Design review of the part built by this model. Coordinates are the model's own, in mm. Face numbers are marked on the shaded views. A direction names the side the tool comes from. Give positions to 0.01 mm unless a question says otherwise; leave off trailing zeros. Write each loop counter-clockwise with the first axis right and the second up, starting at its lowest first coordinate (ties: lowest second). Pieces come first, ordered by that corner, then holes. Notation, with made-up numbers: (62, 8) -> (69, 8) arc R9 cw to (69, 12) -> close; hole circle Ø1 at (-16.5, 87). An arc over 180 degrees is marked (long way). Answer as a JSON object with one key per item and string values.
```python
from build123d import *

# Parameters (mm, degrees)
EXTRUDE_THIN1_DEPTH = 3
CUT_EXTRUDE1_REACH  = 93.341
SKETCH2_R           = 1.25
CUT_EXTRUDE2_REACH  = 93.713
SKETCH3_R           = 1.25
FILLET1_R           = 3


with BuildPart() as part:
    # Sketch1 → Extrude-Thin1 (new, symmetric)
    with BuildSketch(Plane.XY):
        with BuildLine():
            Line((0, 0), (14.004467228, -0.760906267))
            ThreePointArc((14.004467228, -0.760906267), (14.140049985, -0.766428865), (14.275732677, -0.768270184))
            Line((14.275732677, -0.768270184), (60.65, -0.768270184))
            ThreePointArc((60.65, -0.768270184), (62.65, -0.232371799), (64.114101615, 1.231729816))
            Line((64.114101615, 1.231729816), (71.296338964, 13.671729816))
            ThreePointArc((71.296338964, 13.671729816), (72.760440579, 15.135831431), (74.760440579, 15.671729816))
            Line((74.760440579, 15.671729816), (89.99, 15.671729816))
            Line((89.99, 15.671729816), (89.99, 16.671729816))
            Line((89.99, 16.671729816), (74.760440579, 16.671729816))
            ThreePointArc((74.760440579, 16.671729816), (72.260440579, 16.001856835), (70.43031356, 14.171729816))
            Line((70.43031356, 14.171729816), (63.248076211, 1.731729816))
            ThreePointArc((63.248076211, 1.731729816), (62.15, 0.633653605), (60.65, 0.231729816))
            Line((60.65, 0.231729816), (14.275732677, 0.231729816))
            ThreePointArc((14.275732677, 0.231729816), (14.167186524, 0.233202871), (14.058720318, 0.23762095))
            Line((14.058720318, 0.23762095), (0.05425309, 0.998527217))
            Line((0.05425309, 0.998527217), (0, 0))
        make_face()
    extrude(amount=EXTRUDE_THIN1_DEPTH, both=True)

    # Sketch2 → Cut-Extrude1 (cut, up to next)
    with BuildSketch(Plane(origin=(0.054253089686214166, 0.9985272165842555, 0), x_dir=(0.998527216584255, -0.05425308968621415, 0), z_dir=(0.054253089686214145, 0.9985272165842549, 0)), mode=Mode.PRIVATE) as cut_extrude1_sk1:
        with Locations(Location((3, 0, 0), (0, 0, 180))):
            Circle(SKETCH2_R)
    cut_extrude1_tool1 = extrude(cut_extrude1_sk1.sketch, amount=-CUT_EXTRUDE1_REACH, mode=Mode.PRIVATE) & part.part
    add(cut_extrude1_tool1.solids().sort_by_distance((3.049835, 0.835768, 0))[0], mode=Mode.SUBTRACT)

    # Sketch3 → Cut-Extrude2 (cut, up to next)
    with BuildSketch(Plane(origin=(0, 16.671729816, 0), x_dir=(1, 0, 0), z_dir=(0, 1, 0)), mode=Mode.PRIVATE) as cut_extrude2_sk1:
        with Locations(Location((86.99, 0, 0), (0, 0, 270))):
            Circle(SKETCH3_R)
    cut_extrude2_tool1 = extrude(cut_extrude2_sk1.sketch, amount=-CUT_EXTRUDE2_REACH, mode=Mode.PRIVATE) & part.part
    add(cut_extrude2_tool1.solids().sort_by_distance((86.99, 16.67173, 0))[0], mode=Mode.SUBTRACT)

    # Fillet1
    fillet1_edges = [part.edges().sort_by_distance(p)[0] for p in [
        (0.027126545, 0.499263608, -3),
        (0.027126545, 0.499263608, 3),
        (89.99, 16.171729816, -3),
        (89.99, 16.171729816, 3),
    ]]
    fillet(fillet1_edges, radius=FILLET1_R - 0.0001)  # a hair under: the kernel refuses the full size


solid = part.part
```
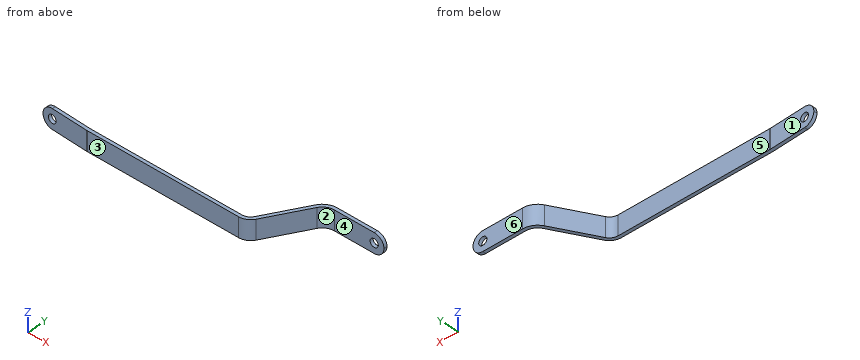
(1) The part is to be moulded in two halves that separate along X. For the marked faces 1, 2 and 3, say which applies: +X half, -X half, draft (parallel to the pull), parting line (faces both ways), or undercut.
Here are the results:
{"face 1": "undercut", "face 2": "+X half", "face 3": "draft"}
(2) For line 1 along Z through (x, y) = (86.99, 16.2); line 2 along Y through (x, z) = (75, 0); line 3 along Y through (x, z) = (33.5, 0), list the stretches that pass through material, from the lowest coordinate up.
Here are the results:
{"line 1": "z = -3 to -1.25, 1.25 to 3", "line 2": "y = 15.67 to 16.67", "line 3": "y = -0.77 to 0.23"}
(3) We need section A-A, the plane z = -2. State the section outline as (x, y) points, then the cut area to 3 significant figures.
Here are the results:
{"outline": "(0.76, -0.04) -> (14, -0.76) arc R5 ccw to (14.28, -0.77) -> (60.65, -0.77) arc R4 ccw to (64.11, 1.23) -> (71.3, 13.67) arc R4 cw to (74.76, 15.67) -> (89.23, 15.67) -> (89.23, 16.67) -> (74.76, 16.67) arc R5 ccw to (70.43, 14.17) -> (63.25, 1.73) arc R3 cw to (60.65, 0.23) -> (14.28, 0.23) arc R4 cw to (14.06, 0.24) -> (0.82, 0.96) -> close", "area": "97.1 mm²"}
(4) We need section B-B, the plane x = 29. State the section outline as (y, z) points, then the cut area to 3 significant figures.
Here are the results:
{"outline": "(-0.77, -3) -> (0.23, -3) -> (0.23, 3) -> (-0.77, 3) -> close", "area": "6.00 mm²"}
(5) We need section D-D, the plane z = 2.25. State the section outline as (x, y) points.
Here are the results:
{"outline": "(1.01, -0.06) -> (14, -0.76) arc R5 ccw to (14.28, -0.77) -> (60.65, -0.77) arc R4 ccw to (64.11, 1.23) -> (71.3, 13.67) arc R4 cw to (74.76, 15.67) -> (88.97, 15.67) -> (88.97, 16.67) -> (74.76, 16.67) arc R5 ccw to (70.43, 14.17) -> (63.25, 1.73) arc R3 cw to (60.65, 0.23) -> (14.28, 0.23) arc R4 cw to (14.06, 0.24) -> (1.07, 0.94) -> close"}
(6) Clearance check with flat-ended pins moving along their axes: pin 1 (4 mm diameter, centred on x = 32.5, y = 2.5, fed in from -Z); pin 2 (1.5 mm diameter, centred on x = 54.5, z = 0, fed in from +Y); pin 3 (3 mm diameter, centred on y = 3, z = -2, fed in from +X); pin 4 (1.8 mm diameter, centred on x = 84.5, z = 0, fed in from -Y). State where each tip first meets the part, or that it passes through.
Here are the results:
{"pin 1": "passes through", "pin 2": "stops at y = 0.23", "pin 3": "stops at x = 66", "pin 4": "stops at y = 15.67"}
(7) For the marked faces 4, 5 and 6, list the 3-axis set-ups (+Z, -Z, +X, -X, +Y, -Y) from which the entire face can be reached by the end or side of a thin tool; tool diameter is ignored.
Here are the results:
{"face 4": "+Z, -Z, +X, -Y", "face 5": "+Z, -Z, +Y", "face 6": "+Z, -Z, +X, -X, +Y"}
(8) We need section C-C, the plane y = 5.5. State the section outline as (x, z) points.
Here are the results:
{"outline": "(65.42, -3) -> (66.58, -3) -> (66.58, 3) -> (65.42, 3) -> close"}
